Read the model definition and answer for the solid it produces. Units are mm, in the model's axes. Round coordinates to 2 decimals unless told otherwise and drop trailing zeros. Order: outer loops, then holes, each group sorted by start corner. A loop starts at its lowest first (then second) coordinate and runs counter-clockwise, first axis right, second up. Notation, with made-up numbers: (10, 12.5) -> (16, 12.5) arc R26 ccw to (16, 27.5) -> close; hole circle Ø3 at (51, 55). An arc over 180 degrees is marked (long way). Use a Markdown table: item, result. Add a question column.
1. Consider L1, parallel to Y at x = 0, z = 5.25 (3 decimals); L2, parallel to X at y = 2.4, z = 14.25; L3, parallel to X at y = 3.35, z = 2. Determine where each line is inside the solid, lowest interval first. Write a range as [from, to].
2. Section A-A, the plane z = 10 is taken. Give the vertices of the cut face in (x, y) (3 decimals), then the cut area to 3 significant figures.
3. Given pin 1 (1 mm diameter, centred on x = -2.5, z = 16.5, fed in from +Y); pin 2 (1.5 mm diameter, centred on y = 1.5, z = 13.5, fed in from -X); pin 3 (1 mm diameter, centred on y = 5, z = 5.5, fed in from +X); pin 4 (1 mm diameter, centred on x = -2, z = 8, fed in from -Y) (3 decimals), each flat-ended and moving along its own axis, determine where each tip first touches the part or whether it passes through.
4. The mould has two halves that part along X. Classify faces 1 (the face through (2.393, 1.819, 9.86)), 2 (the face through (-2.37, 1.78, 9.86)), 3 (the face through (-0.2, 1.69, 9.86)), 4 (the face through (0, 5.925, 10)): +X half, -X half, draft (parallel to the pull), parting line (faces both ways), or undercut.
5. Section D-D, the plane y = 1.4 is taken. Give the vertices of the cut face in (x, z), then the cut area to 3 significant figures.
6. Section C-C, the plane y = 3.95 is taken. Give the vertices of the cut face in (x, z), then the cut area to 3 significant figures.
7. Section B-B, the plane x = 0 is taken. Give the vertices of the cut face in (y, z) (3 decimals).
Autodesk Inventor part; units mm, degrees
ref_plane "YZ Plane" through (0, 0, 0) normal (1, 0, 0) x (0, 1, 0)
ref_plane "XZ Plane" through (0, 0, 0) normal (0, 1, 0) x (-1, 0, 0)
ref_plane "XY Plane" through (0, 0, 0) normal (0, 0, 1) x (1, 0, 0)
sketch "Sketch1" plane through (0, 0, 0) normal (0, 0, 1) x (1, 0, 0)
  arc A0 (-3.175, 3.175) -> (0, 0) centre (0.0002, 3.1752) ccw construction
  line L0 (44.45, 0) -> (0, 0) construction
  arc A1 (44.45, 0) -> (47.625, 3.175) centre (44.4498, 3.1752) ccw construction
  line L1 (47.625, 79.375) -> (47.625, 3.175) construction
  arc A2 (47.625, 79.375) -> (44.45, 82.55) centre (44.4498, 79.3748) ccw construction
  line L2 (0, 82.55) -> (44.45, 82.55) construction
  arc A3 (0, 82.55) -> (-3.175, 79.375) centre (0.0002, 79.3748) ccw construction
  line L3 (-3.175, 3.175) -> (-3.175, 79.375) construction
  circle A4 centre (0, 3.175) radius 1.6 construction
  circle A5 centre (7.112, 4.191) radius 0.51 construction
  circle A6 centre (7.112, 9.271) radius 0.51 construction
  circle A7 centre (7.112, 6.731) radius 0.51 construction
  circle A8 centre (9.652, 6.731) radius 0.51 construction
  circle A9 centre (9.652, 4.191) radius 0.51 construction
  circle A10 centre (9.652, 9.271) radius 0.51 construction
  circle A11 centre (15.655, 10.499) radius 1.15 construction
  circle A12 centre (14.225, 36.449) radius 0.85 construction
  circle A13 centre (4.699, 60.198) radius 0.51 construction
  circle A14 centre (4.699, 57.658) radius 0.51 construction
  circle A15 centre (0, 79.375) radius 1.6 construction
  circle A16 centre (4.699, 62.738) radius 0.51 construction
  circle A17 centre (4.699, 65.278) radius 0.51 construction
  circle A18 centre (13.7, 69.341) radius 0.46 construction
  circle A19 centre (16.2, 69.341) radius 0.46 construction
  circle A20 centre (6.13, 72.051) radius 1.15 construction
  circle A21 centre (11.7, 69.341) radius 0.46 construction
  circle A22 centre (9.2, 69.341) radius 0.46 construction
  circle A23 centre (23.225, 13.209) radius 0.46 construction
  circle A24 centre (25.725, 13.209) radius 0.46 construction
  circle A25 centre (18.725, 13.209) radius 0.46 construction
  circle A26 centre (21.225, 13.209) radius 0.46 construction
  circle A27 centre (28.795, 10.499) radius 1.15 construction
  circle A28 centre (44.45, 3.175) radius 1.6 construction
  circle A29 centre (30.225, 36.449) radius 0.85 construction
  circle A30 centre (39.751, 57.531) radius 0.51 construction
  circle A31 centre (39.751, 60.071) radius 0.51 construction
  circle A32 centre (31.385, 69.341) radius 0.46 construction
  circle A33 centre (33.385, 69.341) radius 0.46 construction
  circle A34 centre (19.27, 72.051) radius 1.15 construction
  circle A35 centre (28.885, 69.341) radius 0.46 construction
  circle A36 centre (25.815, 72.051) radius 1.15 construction
  circle A37 centre (39.751, 65.151) radius 0.51 construction
  circle A38 centre (39.751, 62.611) radius 0.51 construction
  circle A39 centre (35.885, 69.341) radius 0.46 construction
  circle A40 centre (38.955, 72.051) radius 1.15 construction
  circle A41 centre (44.45, 79.375) radius 1.6 construction
  circle A42 centre (0, 3.175) radius 1.5
  circle A43 centre (0, 3.175) radius 2.75 construction
  line L4 (1.5877, 0.425) -> (-1.5877, 0.425)
  line L5 (-1.5877, 0.425) -> (-3.1754, 3.175)
  line L6 (-3.1754, 3.175) -> (-1.5877, 5.925)
  line L7 (-1.5877, 5.925) -> (1.5877, 5.925)
  line L8 (1.5877, 5.925) -> (3.1754, 3.175)
  line L9 (3.1754, 3.175) -> (1.5877, 0.425)
  dimension "d0" = 3
  dimension "d1" = 5.5
extrude "Extrusion1" add sketch "Sketch1" along normal blind 20
properties part number "Standoff"
Verdict:
| question | item | result |
|---|---|---|
| 1 | L1 | y = [0.425, 1.675], [4.675, 5.925] |
| 1 | L2 | x = [-2.73, -1.28], [1.28, 2.73] |
| 1 | L3 | x = [-3.07, -1.49], [1.49, 3.07] |
| 2 | outline | (-3.175, 3.175) -> (-1.588, 0.425) -> (1.588, 0.425) -> (3.175, 3.175) -> (1.588, 5.925) -> (-1.588, 5.925) -> close; hole circle Ø3 at (0, 3.175) |
| 2 | area | 19.1 mm2 |
| 3 | pin 1 | stops at y = 5.21 |
| 3 | pin 2 | stops at x = -2.64 |
| 3 | pin 3 | stops at x = 2.41 |
| 3 | pin 4 | stops at y = 0.425 |
| 4 | face 1 | +X half |
| 4 | face 2 | -X half |
| 4 | face 3 | undercut |
| 4 | face 4 | draft |
| 5 | outline | (-2.15, 0) -> (2.15, 0) -> (2.15, 20) -> (-2.15, 20) -> close |
| 5 | area | 86.0 mm2 |
| 6 | outline | (-2.73, 0) -> (-1.28, 0) -> (-1.28, 20) -> (-2.73, 20) -> close; (1.28, 0) -> (2.73, 0) -> (2.73, 20) -> (1.28, 20) -> close |
| 6 | area | 57.7 mm2 |
| 7 | outline | (0.425, 0) -> (1.675, 0) -> (1.675, 20) -> (0.425, 20) -> close; (4.675, 0) -> (5.925, 0) -> (5.925, 20) -> (4.675, 20) -> close |
